Part model, mm, in its own coordinate system. A direction names the side the tool comes from. Give positions to 0.01 mm unless a question says otherwise; leave off trailing zeros. Order: outer loops, then holes, each group sorted by start corner. A loop starts at its lowest first (then second) coordinate and runs counter-clockwise, first axis right, second up. Notation, with made-up numbers: (39.5, 5) - (46.5, 5) arc R26 cw to (46.5, 29) - close; hole circle Ø9 at (82, -4.5). An arc over 180 degrees is marked (long way). One line per item, written item: value.
Autodesk Inventor part; units mm, degrees
ref_plane "YZ Plane" through (0, 0, 0) normal (1, 0, 0) x (0, 1, 0)
ref_plane "XZ Plane" through (0, 0, 0) normal (0, 1, 0) x (-1, 0, 0)
ref_plane "XY Plane" through (0, 0, 0) normal (0, 0, 1) x (1, 0, 0)
sketch "Sketch1" plane through (0, 0, 0) normal (0, 0, 1) x (1, 0, 0)
  line L0 (0, 0) -> (28.2, 0)
  line L1 (28.2, 0) -> (28.2, 30.2)
  line L2 (28.2, 30.2) -> (0, 30.2)
  line L3 (0, 30.2) -> (0, 0)
  line L4 (14.1, 30.2) -> (14.1, 0)
  line L5 (31.1, -1.9) -> (-2.9, -1.9)
  line L6 (-2.9, -1.9) -> (-2.9, 32.1)
  line L7 (-2.9, 32.1) -> (31.1, 32.1)
  line L8 (31.1, 32.1) -> (31.1, -1.9)
  line L9 (31.1, -1.9) -> (-2.9, 32.1) construction
  line L10 (-2.9, -1.9) -> (31.1, 32.1) construction
  point P0 (14.1, 15.1)
  dimension "d0" = 30.2
  dimension "d1" = 28.2
  dimension "d2" = 34
  dimension "d3" = 34
extrude "Extrusion1" add sketch "Sketch1" along normal blind 0.8
fillet "Fillet1" radius 3 4 edges at (0, 0, 0.4) (0, 30.2, 0.4) (28.2, 30.2, 0.4) (28.2, 0, 0.4)
fillet "Fillet2" radius 5 4 edges at (31.1, 32.1, 0.4) (-2.9, 32.1, 0.4) (31.1, -1.9, 0.4) (-2.9, -1.9, 0.4)
fillet "Fillet3" radius 0.2 24 edges at (-1.4355, 30.6355, 0) (-2.9, 15.1, 0) (-1.4355, -0.4355, 0) (14.1, -1.9, 0) (29.6355, -0.4355, 0) (31.1, 15.1, 0) (29.6355, 30.6355, 0) (14.1, 32.1, 0) (14.1, 32.1, 0.8) (29.6355, 30.6355, 0.8) (31.1, 15.1, 0.8) (29.6355, -0.4355, 0.8) (14.1, -1.9, 0.8) (-1.4355, -0.4355, 0.8) (-2.9, 15.1, 0.8) (-1.4355, 30.6355, 0.8) (0, 15.1, 0.8) (14.1, 0, 0.8) (28.2, 15.1, 0.8) (14.1, 30.2, 0.8) (14.1, 30.2, 0) (28.2, 15.1, 0) (14.1, 0, 0) (0, 15.1, 0)
properties part number "LeptonBlockSpacer"
1) Slice it at A-A on y = 5.5. Write the cut outline in (x, z), then the cut area to 3 significant figures.
Answer:
outline: (-2.9, 0.2) arc R0.2 ccw to (-2.7, 0) - (-0.2, 0) arc R0.2 ccw to (0, 0.2) - (0, 0.6) arc R0.2 ccw to (-0.2, 0.8) - (-2.7, 0.8) arc R0.2 ccw to (-2.9, 0.6) - close; (28.2, 0.2) arc R0.2 ccw to (28.4, 0) - (30.9, 0) arc R0.2 ccw to (31.1, 0.2) - (31.1, 0.6) arc R0.2 ccw to (30.9, 0.8) - (28.4, 0.8) arc R0.2 ccw to (28.2, 0.6) - close
area: 4.57 mm2
2) Which spindle directions (+Z, -Z, +X, -X, +Y, -Y) get a long thin tool onto all of the face, cutting with end or side? Do faces 4 (the face through (27.3, 0.86, 0.4)), 5 (the face through (29.67, 30.6, 0.4)). Say none if no direction does.
Answer:
face 4: +Z, -Z
face 5: +Z, -Z, +X, +Y
3) Two-plate mould, pull along Y, no slides. Class faces 1 (the face through (-1, 14, 0)), 2 (the face through (27.34, 29.3, 0.4)), 3 (the face through (-1.47, -0.4, 0.4)): pulls with the +Y half, pulls with the -Y half, needs draft (parallel to the pull), parting line crosses it, or undercut.
Answer:
face 1: needs draft
face 2: undercut
face 3: pulls with the -Y half
4) Wall check: line 1 along X through (y, z) = (4.5, 0.2); line 2 along Y through (x, z) = (19, 0.45); line 3 along Y through (x, z) = (1, 0.25). Give the ranges that are in metal, low to high. Write a range as [from, to].
Answer:
line 1: x = [-2.9, 0], [28.2, 31.1]
line 2: y = [-1.9, 0], [30.2, 32.1]
line 3: y = [-1.78, 0.76], [29.44, 31.98]
5) Slice it at B-B on x = 4. Write the cut outline in (y, z), then the cut area to 3 significant figures.
Answer:
outline: (-1.9, 0.2) arc R0.2 ccw to (-1.7, 0) - (-0.2, 0) arc R0.2 ccw to (0, 0.2) - (0, 0.6) arc R0.2 ccw to (-0.2, 0.8) - (-1.7, 0.8) arc R0.2 ccw to (-1.9, 0.6) - close; (30.2, 0.2) arc R0.2 ccw to (30.4, 0) - (31.9, 0) arc R0.2 ccw to (32.1, 0.2) - (32.1, 0.6) arc R0.2 ccw to (31.9, 0.8) - (30.4, 0.8) arc R0.2 ccw to (30.2, 0.6) - close
area: 2.97 mm2
6) Slice it at C-C on z = 0.35. Write the cut outline in (x, y).
Answer:
outline: (-2.9, 3.1) arc R5 ccw to (2.1, -1.9) - (26.1, -1.9) arc R5 ccw to (31.1, 3.1) - (31.1, 27.1) arc R5 ccw to (26.1, 32.1) - (2.1, 32.1) arc R5 ccw to (-2.9, 27.1) - close; hole (0, 3) arc R3 ccw to (3, 0) - (25.2, 0) arc R3 ccw to (28.2, 3) - (28.2, 27.2) arc R3 ccw to (25.2, 30.2) - (3, 30.2) arc R3 ccw to (0, 27.2) - close
